Build history of the part. All positions in model axes, mm. A direction names the side the tool comes from. Coordinates: 2 decimals unless noted, no trailing zeros. Order: outer loops, then holes, each group sorted by start corner. A loop starts at its lowest first (then second) coordinate and runs counter-clockwise, first axis right, second up. Notation, with made-up numbers: M -8,-14.5 L 24,-14.5 A15 cw 24,-8.5 Z; hole C 41.5,-18.5 d4. An arc over 180 degrees is marked long. Use a Markdown table: item, result. Add a question column.
from build123d import *

# Parameters (mm, degrees)
F0_W         = 609.6
F0_H         = 381
F1_DEPTH     = 635
F2_DEPTH     = 25.4
F3_W         = 50.8
F3_H         = 76.2
F3_W_2       = 406.4
F4_DEPTH     = 1574.8
F5_W         = 50.8
F5_H         = 76.2
F5_W_2       = 203.2
F6_DEPTH     = 970.28
F7_W         = 25.4
F7_H         = 379.8168087482
F8_DEPTH     = 25.4
F9_R         = 12.7
F10_T1_DEPTH = 459.0207478943
F10_T3_DEPTH = 674.9207478943


# Not quite as in the source:
# - a fillet or chamfer that OpenCascade refuses, or shapes differently, is made with other operations: its cross-section is extruded or revolved along the edge and cut away or added


with BuildPart() as f1:
    # F0 (on Top) → F1 (new body)
    with BuildSketch(Plane.XY):
        with Locations((304.8, 190.5)):
            Rectangle(F0_W, F0_H)
    extrude(amount=F1_DEPTH)

    # F2 (add): a face of the model
    f2_faces = [f1.faces().sort_by_distance(p)[0] for p in [
        (304.8, 0, 317.5),
    ]]
    extrude(f2_faces, amount=F2_DEPTH)

    # F3 (on face) → F4 (cut)
    with BuildSketch(Plane.XZ.offset(25.4)):
        with Locations((25.4, 38.1)):
            Rectangle(F3_W, F3_H)
        with Locations((304.8, 38.1)):
            Rectangle(F3_W_2, F3_H)
        with Locations((584.2, 38.1)):
            Rectangle(F3_W, F3_H)
    extrude(amount=-F4_DEPTH, mode=Mode.SUBTRACT)

    # F5 (on face) → F6 (cut)
    with BuildSketch(Plane.YZ.offset(558.8)):
        with Locations((0, 38.1)):
            Rectangle(F5_W, F5_H)
        with Locations((177.8, 38.1)):
            Rectangle(F5_W_2, F5_H)
        with Locations((355.6, 38.1)):
            Rectangle(F5_W, F5_H)
    extrude(amount=-F6_DEPTH, mode=Mode.SUBTRACT)

    # F7 (on face) → F8 (cut)
    with BuildSketch(Plane.XZ.offset(25.4)):
        with Locations((292.1, 266.1084043741)):
            Rectangle(F7_W, F7_H)
        Polygon((609.6, 481.4168087482), (0, 481.4168087482), (0, 456.0168087482), (279.4, 456.0168087482), (304.8, 456.0168087482), (609.6, 456.0168087482), align=None)
    extrude(amount=-F8_DEPTH, mode=Mode.SUBTRACT)

    # F9
    f9_edges = [f1.edges().sort_by_distance(p)[0] for p in [
        (609.6, -25.4, 558.208404),
        (304.8, -25.4, 635),
        (0, -25.4, 558.208404),
        (304.8, -25.4, 481.416809),
        (279.4, -25.4, 266.108404),
        (139.7, -25.4, 456.016809),
        (0, -25.4, 266.108404),
        (139.7, -25.4, 76.2),
        (609.6, -25.4, 266.108404),
        (457.2, -25.4, 456.016809),
        (304.8, -25.4, 266.108404),
        (457.2, -25.4, 76.2),
    ]]
    fillet(f9_edges, radius=F9_R)

    # F10: chamfer of 12.7 on 4 edges, made by hand

    # F10_s2 → F10_t1 (cut)
    with BuildSketch(Plane.XZ.offset(-413.6603739472)):
        Polygon((0, 622.3), (12.7, 635), (0, 635), align=None)
        Polygon((596.9, 635), (609.6, 622.3), (609.6, 635), align=None)
    extrude(amount=F10_T1_DEPTH, mode=Mode.SUBTRACT)

    # F10_s4 → F10_t3 (cut)
    with BuildSketch(Plane.YZ.offset(-32.6603739472)):
        Polygon((381, 622.3), (368.3, 635), (381, 635), align=None)
    extrude(amount=F10_T3_DEPTH, mode=Mode.SUBTRACT)


solid = f1.part
(1) Drop flat-ended pins along their axis: P1, Ø5, axis at x = 485, y = 190.5, coming from the -Z side; P2, Ø10, axis at y = 340, z = 218, coming from the -X side; P3, Ø15, axis at x = 543.5, z = 45, coming from the -Y side. Give the stop position or say it passes through.
(2) Drill centre lines: line 1 along Z through (x, y) = (222, -5.5); line 2 along Z through (x, y) = (562, 119.5). Where is each one in solid material? Low to high. Write a range as from..to.
(3) Mould opens along Y. For faces 5 (the flat face through (77, 25.4, 38)), 6 (the flat face through (534, 76.2, 38)), 7 (the flat face through (558.8, 50, 38)), 8 (the flat face through (77, 76.2, 38)) say: released by +Y, released by -Y, zero draft, split by the parting line, or undercut.
(4) Which spindle directions (+Z, -Z, +X, -X, +Y, -Y) get a long thin tool onto all of the face, cutting with end or side? Do faces 1 (the flat face through (534, 279.4, 38)), 2 (the flat face through (558.8, 304, 38)), 3 (the flat face through (50.8, 304, 38)), 4 (the flat face through (101.6, 304, 38)). Say none if no direction does.
(5) Slice it at B-B on y = 258. Give the cut face in (x, z), and give its area (3 significant figures).
(6) Slice it at A-A on x = 413. Give the cut face in (y, z).
Solutions:
| question | item | result |
|---|---|---|
| 1 | P1 | z = 76.2 |
| 1 | P2 | x = 0 |
| 1 | P3 | y = 25.4 |
| 2 | line 1 | 76.2..456.02, 481.42..635 |
| 2 | line 2 | 76.2..635 |
| 3 | face 5 | released by -Y |
| 3 | face 6 | undercut |
| 3 | face 7 | zero draft |
| 3 | face 8 | undercut |
| 4 | face 1 | -Z, +X, -X |
| 4 | face 2 | -Z, +X, +Y, -Y |
| 4 | face 3 | -Z, -X, +Y, -Y |
| 4 | face 4 | -Z, +Y, -Y |
| 5 | outline | M 0,76.2 L 609.6,76.2 L 609.6,622.3 L 596.9,635 L 12.7,635 L 0,622.3 Z |
| 5 | area | 340,000 mm² |
| 6 | outline | M -25.4,88.9 A12.7 ccw -12.7,76.2 L 381,76.2 L 381,622.3 L 368.3,635 L -12.7,635 A12.7 ccw -25.4,622.3 L -25.4,494.12 A12.7 ccw -12.7,481.42 L 0,481.42 L 0,456.02 L -12.7,456.02 A12.7 ccw -25.4,443.32 Z |
